from build123d import *

# Parameters (mm, degrees)
F0_W        = 76.2
F0_H        = 50.8
F1_DEPTH    = 25.4
F2_W        = 15.6074212864
F2_H        = 14.8792807013
F3_DEPTH    = 25.4
F4_R        = 5.08
F5_T        = 2.54
F5_T3_DEPTH = 30.48


# Not quite as in the source:
# - a shell that OpenCascade refuses in one call is made with other operations: the cavity is built on its own and cut out


with BuildPart() as f1:
    # F0 (on Top) → F1 (new body)
    with BuildSketch(Plane.XY):
        with Locations((38.1, 25.4)):
            Rectangle(F0_W, F0_H)
    extrude(amount=F1_DEPTH)

    # F2 (on face) → F3 (cut, through all)
    with BuildSketch(Plane.XY.offset(25.4)):
        with Locations((19.1314755939, 19.2197160795)):
            Rectangle(F2_W, F2_H)
    extrude(amount=-F3_DEPTH, mode=Mode.SUBTRACT)

    # F4
    f4_edges = [f1.edges().sort_by_distance(p)[0] for p in [
        (38.1, 0, 25.4),
        (76.2, 0, 12.7),
        (76.2, 50.8, 12.7),
        (76.2, 25.4, 0),
        (76.2, 25.4, 25.4),
        (0, 0, 12.7),
        (0, 25.4, 25.4),
    ]]
    fillet(f4_edges, radius=F4_R)

    # F5: shell of thickness 2.54, made by hand


with BuildPart() as f5_core1:
    # F5_t2: copy of F1
    add(f1.part)

    # the walls: a layer under each face that stays
    f5_faces = [f5_core1.faces().sort_by_distance(p)[0] for p in [
        (0, 27.94, 10.16),
        (35.56, 50.8, 12.7),
        (1.4878975516, 27.94, 23.9121024484),
        (1.4878975516, 1.4878975516, 10.16),
        (38.1, 27.94, 25.4),
        (74.7121026222, 49.3121022747, 12.7),
        (1.4878975516, 2.54, 22.86),
        (38.1, 0, 10.16),
        (74.7121025744, 25.4, 1.4878976776),
        (11.3277649507, 19.2197160795, 12.7),
        (19.1314755939, 11.7800757289, 12.7),
        (26.9351862371, 19.2197160795, 12.7),
        (19.1314755939, 26.6593564302, 12.7),
        (74.7121026222, 27.94, 23.9121022747),
        (38.1, 1.4878975516, 23.9121024484),
        (76.2, 25.4, 12.7),
        (74.7121024484, 1.4878975516, 10.16),
        (74.7121024484, 2.54, 22.86),
    ]]
    thicken(f5_faces, amount=-F5_T, mode=Mode.SUBTRACT)

    # F5_s4 → F5_t3 (cut)
    with BuildSketch(Plane.XY.offset(-2.54)):
        Polygon((11.3531649507, 26.6339564302), (8.7877649507, 26.6593564302), (8.7877649507, 29.1993564302), (11.3277649507, 29.1993564302), align=None)
        Polygon((11.3531649507, 11.8054757289), (8.7877649507, 11.7800757289), (8.7877649507, 9.2400757289), (11.3277649507, 9.2400757289), align=None)
        Polygon((26.9097862371, 11.8054757289), (26.9351862371, 9.2400757289), (29.4751862371, 9.2400757289), (29.4751862371, 11.7800757289), align=None)
        Polygon((26.9097862371, 26.6339564302), (29.4751862371, 26.6593564302), (29.4751862371, 29.1993564302), (26.9351862371, 29.1993564302), align=None)
    extrude(amount=F5_T3_DEPTH, mode=Mode.SUBTRACT)


with BuildPart() as f1_1:
    add(f1.part)

    # what is left inside the walls is the cavity
    f5_cavity = [f5_core1.part.solids().sort_by_distance(p)[0] for p in [
        (36.83, 17.78, 0.0254),
    ]]
    add(f5_cavity, mode=Mode.SUBTRACT)


solid = f1_1.part
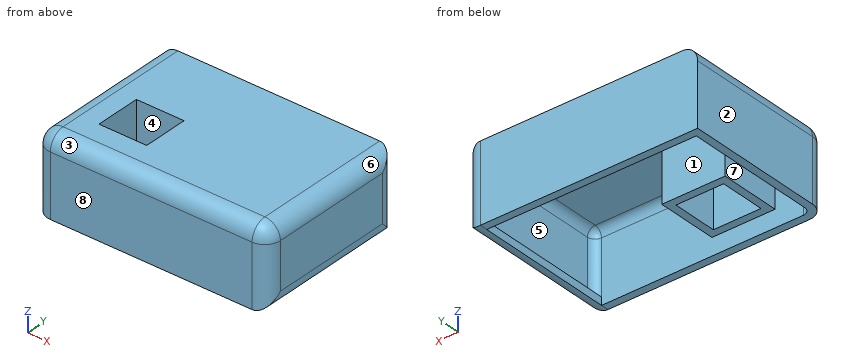
Build history of the part. All positions in model axes, mm. Face numbers are marked on the shaded views. A direction names the side the tool comes from. Give positions to 0.01 mm unless a question says otherwise; leave off trailing zeros. Order: outer loops, then holes, each group sorted by start corner. A loop starts at its lowest first (then second) coordinate and runs counter-clockwise, first axis right, second up. Notation, with made-up numbers: M 23.5,-12.5 L 48.5,-12.5 A6 ccw 48.5,-8.5 Z; hole C 30.5,0.5 d5. An arc over 180 degrees is marked long. Use one line per item in the form item = value.
1) Tool access for the marked faces 4, 5, 6, 7 and 8: list every direction of +Z, -Z, +X, -X, +Y, -Y with a clear straight run to the whole face (end or side of a thin tool).
Calculated:
face_4 = +Z, -Z
face_5 = none
face_6 = +Z, +X, +Y, -Y
face_7 = -Z
face_8 = +Z, -Z, +X, -X, -Y
2) Probe probe 1 along X at (y, z) = (24.5, 15.25); probe 2 along X at (y, z) = (27.5, 20.5); probe 3 along Y at (x, z) = (39, 18.25). List the from-to ranges inside material, lowest first.
Calculated:
probe_1 = 0 to 2.54, 8.79 to 11.33, 26.94 to 29.48, 73.66 to 76.2
probe_2 = 0 to 2.55, 8.79 to 29.48, 73.65 to 76.2
probe_3 = 0 to 2.54, 48.26 to 50.8
3) Saw through at D-D (x = 8). Give the cut face in (y, z), plus the area to 3 significant figures.
Calculated:
outline = M 0,0 L 2.54,0 L 2.54,20.32 A2.54 cw 5.08,22.86 L 48.26,22.86 L 48.26,0 L 50.8,0 L 50.8,25.4 L 5.08,25.4 A5.08 ccw 0,20.32 Z
area = 241 mm2
4) Saw through at B-B (x = 22.5). Give the cut face in (y, z).
Calculated:
outline = M 0,0 L 2.54,0 L 2.54,20.32 A2.54 cw 5.08,22.86 L 9.24,22.86 L 9.24,0 L 11.78,0 L 11.78,25.4 L 5.08,25.4 A5.08 ccw 0,20.32 Z; M 26.66,0 L 29.2,0 L 29.2,22.86 L 48.26,22.86 L 48.26,0 L 50.8,0 L 50.8,25.4 L 26.66,25.4 Z
5) Saw through at A-A (z = 15). Give the cut face in (x, y), plus the area to 3 significant figures.
Calculated:
outline = M 0,5.08 A5.08 ccw 5.08,0 L 71.12,0 A5.08 ccw 76.2,5.08 L 76.2,45.72 A5.08 ccw 71.12,50.8 L 0,50.8 Z; M 8.79,9.24 L 29.48,9.24 L 29.48,29.2 L 8.79,29.2 Z; hole M 2.54,5.08 A2.54 ccw 5.08,2.54 L 71.12,2.54 A2.54 ccw 73.66,5.08 L 73.66,45.72 A2.54 ccw 71.12,48.26 L 2.54,48.26 Z; hole M 11.33,11.78 L 26.94,11.78 L 26.94,26.66 L 11.33,26.66 Z
area = 788 mm2
6) Saw through at C-C (y = 20). Give the cut face in (x, z).
Calculated:
outline = M 0,0 L 2.54,0 L 2.54,20.32 A2.54 cw 5.08,22.86 L 8.79,22.86 L 8.79,0 L 11.33,0 L 11.33,25.4 L 5.08,25.4 A5.08 ccw 0,20.32 Z; M 26.94,0 L 29.48,0 L 29.48,22.86 L 71.12,22.86 A2.54 cw 73.66,20.32 L 73.66,5.08 A2.54 cw 71.12,2.54 L 71.12,0 A5.08 ccw 76.2,5.08 L 76.2,20.32 A5.08 ccw 71.12,25.4 L 26.94,25.4 Z
7) Two-plate mould, pull along X, no slides. Class the marked faces 1, 2 and 3: released by +X, released by -X, zero draft, split by the parting line, or undercut.
Calculated:
face_1 = undercut
face_2 = released by -X
face_3 = zero draft
